Could you check a few things on this model? Use its own coordinates, in mm. Face numbers are marked on the shaded views. Give positions to 0.01 mm unless a question says otherwise; leave off trailing zeros. Loops run counter-clockwise (first coordinate to the right, second up) from the corner with the lowest first, then second, coordinate; pieces in that order, holes last. Notation, with made-up numbers: M -5,76.5 L 41,76.5 A20 ccw 41,112.5 Z; hole C 5.25,71 d4. An arc over 180 degrees is marked long. Answer in a Markdown table with one row per item. Add a question column.
1. If we section it at C-C on y = -14.75: List the corners of the cut face in (x, z) for me, then the cut area to 3 significant figures.
2. I'm going to push flat-ended pins straight in: pin 1 Ø5 at (y, z) = (-3.5, 16) entering from +X; pin 2 Ø3 at (y, z) = (-6.5, 12.5) entering from +X; pin 3 Ø5 at (x, z) = (11, 33) entering from -Y. Where does each tip first touch, or does it pass through?
3. Thinking about a two-plate mould opening in Z: for the marked faces 1, 2 and 3, which applies, released by +Z, released by -Z, zero draft, split by the parting line, or undercut?
4. I need wall thicknesses on line 1 along Z through (x, y) = (0, -13.75); line 2 along X through (y, z) = (-4.75, -19.5); line 3 along X through (y, z) = (-3.75, 23). Which ranges of each line are inside material? Lowest first, please. Write a range as from..to.
5. If we section it at B-B on z = 0: List the corners of the cut face in (x, y) for me, then the cut area to 3 significant figures.
6. If we section it at A-A on x = 0: List the corners of the cut face in (y, z) for me.
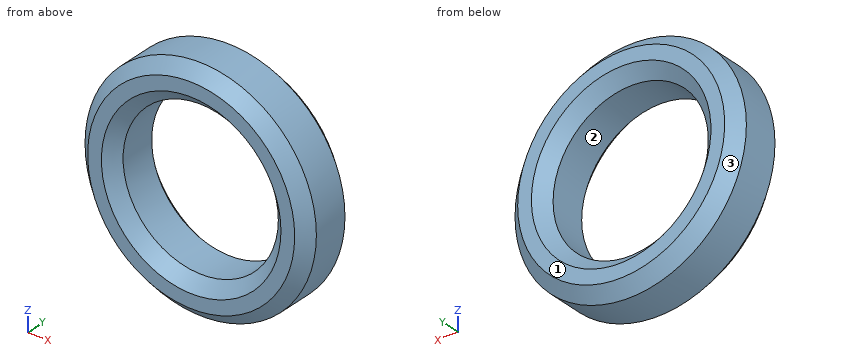
```python
from build123d import *

# Parameters (mm, degrees)
F0_R     = 48.302037
F0_R_2   = 32.411145
F1_DEPTH = 25.4
F2_SIZE  = 5.08


with BuildPart() as f1:
    # F0 (on Front) → F1 (new body)
    with BuildSketch(Plane.XZ):
        Circle(F0_R)
        Circle(F0_R_2, mode=Mode.SUBTRACT)
    extrude(amount=F1_DEPTH)

    # F2
    f2_edges = [f1.edges().sort_by_distance(p)[0] for p in [
        (-48.302037, -25.4, 0),
        (-48.302037, 0, 0),
        (-32.411145, 0, 0),
        (32.411145, -12.7, 0),
        (-32.411145, -25.4, 0),
    ]]
    chamfer(f2_edges, length=F2_SIZE)


solid = f1.part
```
Results:
| question | item | result |
|---|---|---|
| 1 | outline | C 0,0 d96.6; hole C 0,0 d64.82 |
| 1 | area | 4,030 mm2 |
| 2 | pin 1 | x = 46.21 |
| 2 | pin 2 | x = 47.03 |
| 2 | pin 3 | y = -25.19 |
| 3 | face 1 | zero draft |
| 3 | face 2 | undercut |
| 3 | face 3 | split by the parting line |
| 4 | line 1 | -48.3..-32.41, 32.41..48.3 |
| 4 | line 2 | -43.83..-26.3, 26.3..43.83 |
| 4 | line 3 | -40.96..-24.69, 24.69..40.96 |
| 5 | outline | M -48.3,-20.32 L -43.22,-25.4 L -37.49,-25.4 L -32.41,-20.32 L -32.41,-5.08 L -37.49,0 L -43.22,0 L -48.3,-5.08 Z; M 32.41,-20.32 L 37.49,-25.4 L 43.22,-25.4 L 48.3,-20.32 L 48.3,-5.08 L 43.22,0 L 37.49,0 L 32.41,-5.08 Z |
| 5 | area | 704 mm2 |
| 6 | outline | M -25.4,-43.22 L -20.32,-48.3 L -5.08,-48.3 L 0,-43.22 L 0,-37.49 L -5.08,-32.41 L -20.32,-32.41 L -25.4,-37.49 Z; M -25.4,37.49 L -20.32,32.41 L -5.08,32.41 L 0,37.49 L 0,43.22 L -5.08,48.3 L -20.32,48.3 L -25.4,43.22 Z |
